Source: CAD feature listing. Evaluate the final solid. Frame: model axes, mm. A direction names the side the tool comes from. Give positions to 0.01 mm unless a question says otherwise; leave off trailing zeros. Order: outer loops, then holes, each group sorted by start corner. A loop starts at its lowest first (then second) coordinate and runs counter-clockwise, first axis right, second up.
1) First-contact query: P1, Ø5, axis at x = -6.5, y = 36.5, coming from the +Z side; P2, Ø2, axis at x = 15.5, y = 22.5, coming from the +Z side. Flat tips, straight axial feed; report the tip coordinate or a pass-through.
2) Section B-B, the plane z = 21. Return loops of the section in (x, y).
3) Section A-A, the plane x = -31.75. Return loops of the section in (y, z) (3 decimals), plus the area to 3 significant figures.
4) Section C-C, the plane z = 11.5. Return loops of the section in (x, y).
5) Material intervals for line 1 (Y direction, x = -6.35, z = 40.25); line 2 (Y direction, x = -6, z = 41); line 3 (Y direction, x = -1, z = 1), sorted ascending.
6) Section D-D, the plane y = -2.54. Return loops of the section in (x, z), plus the area to 3 significant figures.
7) Draft query along Z for faces 4 (the face through (-35, 13.2, 17.5)), 5 (the face through (-1, 22, -2.54)), 6 (the face through (46.99, 21, 20)). Return one class per face: released by +Z, released by -Z, zero draft, split by the parting line, or undercut.
8) Access query for faces 1 (the face through (25, 42.418, 21)), 2 (the face through (-50.8, 21, 20)), 3 (the face through (-36, 39.878, 21)). Directions: +Z, -Z, +X, -X, +Y, -Y. A direction counts if a zero-diameter tool reaches every point of the face in a straight line with its end or side. Return the directions, or none.
```python
from build123d import *

# Parameters (mm, degrees)
SKETCH1_W           = 97.79
SKETCH1_H           = 67.818
BOSS_EXTRUDE1_DEPTH = 42.418
SKETCH2_W           = 97.79
SKETCH2_H           = 67.818
BOSS_EXTRUDE2_DEPTH = 2.54
SKETCH3_R           = 4.064
CUT_EXTRUDE1_DEPTH  = 68.818
SKETCH4_R           = 5
CUT_EXTRUDE2_DEPTH  = 6.35
SKETCH5_R           = 5.1
CUT_EXTRUDE3_DEPTH  = 15.24
FILLET1_R           = 3.81


with BuildPart() as part:
    # Sketch1 → Boss-Extrude1 (new body)
    with BuildSketch(Plane.XY):
        with Locations((-1.905, 21.209)):
            Rectangle(SKETCH1_W, SKETCH1_H)
        Polygon((7.62, 30.734), (7.62, 42.418), (41.91, 42.418), (41.91, 0), (7.62, 0), (7.62, 11.684), (-16.51, 11.684), (-16.51, 30.734), align=None, mode=Mode.SUBTRACT)
    extrude(amount=BOSS_EXTRUDE1_DEPTH)

    # Sketch2 → Boss-Extrude2 (add)
    with BuildSketch(Plane(origin=(0, 0, 0), x_dir=(-1, 0, 0), z_dir=(0, 0, -1))):
        with Locations((1.905, 21.209)):
            Rectangle(SKETCH2_W, SKETCH2_H)
    extrude(amount=BOSS_EXTRUDE2_DEPTH)

    # Sketch3 → Cut-Extrude1 (cut, through all)
    with BuildSketch(Plane.XZ.offset(12.7)):
        with Locations((-31.75, 19.939)):
            Circle(SKETCH3_R)
    extrude(amount=-CUT_EXTRUDE1_DEPTH, mode=Mode.SUBTRACT)

    # Sketch4 → Cut-Extrude2 (cut)
    with BuildSketch(Plane.XY.offset(42.418)):
        with Locations((-6.35, 37.96)):
            Circle(SKETCH4_R)
        with Locations((-6.35, -2.54)):
            Circle(SKETCH4_R)
    extrude(amount=-CUT_EXTRUDE2_DEPTH, mode=Mode.SUBTRACT)

    # Sketch5 → Cut-Extrude3 (cut)
    with BuildSketch(Plane(origin=(0, 55.118, 0), x_dir=(1, 0, 0), z_dir=(0, 1, 0))):
        with Locations((-31.75, -19.939)):
            Circle(SKETCH5_R)
    extrude(amount=-CUT_EXTRUDE3_DEPTH, mode=Mode.SUBTRACT)

    # Fillet1
    fillet1_edges = [part.edges().sort_by_distance(p)[0] for p in [
        (46.99, 21.209, 42.418),
        (46.99, 21.209, -2.54),
        (-50.8, 21.209, -2.54),
        (-50.8, 21.209, 42.418),
    ]]
    fillet(fillet1_edges, radius=FILLET1_R)


solid = part.part
```
From the geometry:
1. P1: stops at z = 36.07
1. P2: stops at z = 0
2. outline: (-50.8, -12.7) - (-35.67, -12.7) - (-35.67, 39.88) - (-36.74, 39.88) - (-36.74, 55.12) - (-50.8, 55.12) - close; (-27.83, -12.7) - (46.99, -12.7) - (46.99, 55.12) - (-26.76, 55.12) - (-26.76, 39.88) - (-27.83, 39.88) - close; hole (-16.51, 11.68) - (7.62, 11.68) - (7.62, 0) - (41.91, 0) - (41.91, 42.42) - (7.62, 42.42) - (7.62, 30.73) - (-16.51, 30.73) - close
3. outline: (-12.7, -2.54) - (55.118, -2.54) - (55.118, 14.839) - (39.878, 14.839) - (39.878, 15.875) - (-12.7, 15.875) - close; (-12.7, 24.003) - (39.878, 24.003) - (39.878, 25.039) - (55.118, 25.039) - (55.118, 42.418) - (-12.7, 42.418) - close
3. area: 2,470 mm2
4. outline: (-50.8, -12.7) - (46.99, -12.7) - (46.99, 55.12) - (-50.8, 55.12) - close; hole (-16.51, 11.68) - (7.62, 11.68) - (7.62, 0) - (41.91, 0) - (41.91, 42.42) - (7.62, 42.42) - (7.62, 30.73) - (-16.51, 30.73) - close
5. line 1: y = -12.7 to -7.54, 2.46 to 11.68, 30.73 to 32.96, 42.96 to 55.12
5. line 2: y = -12.7 to -7.53, 2.45 to 11.68, 30.73 to 32.97, 42.95 to 55.12
5. line 3: y = -12.7 to 11.68, 30.73 to 55.12
6. outline: (-50.8, 1.27) arc R3.81 ccw to (-46.99, -2.54) - (43.18, -2.54) arc R3.81 ccw to (46.99, 1.27) - (46.99, 38.61) arc R3.81 ccw to (43.18, 42.42) - (-1.35, 42.42) - (-1.35, 36.07) - (-11.35, 36.07) - (-11.35, 42.42) - (-46.99, 42.42) arc R3.81 ccw to (-50.8, 38.61) - close; hole circle Ø8.13 at (-31.75, 19.94)
6. area: 4,270 mm2
7. face 4: undercut
7. face 5: released by -Z
7. face 6: zero draft
8. face 1: +Z
8. face 2: +Z, -Z, -X, +Y, -Y
8. face 3: +Y
